Build history of the part. All positions in model axes, mm. Face numbers are marked on the shaded views. A direction names the side the tool comes from. Give positions to 0.01 mm unless a question says otherwise; leave off trailing zeros. Loops run counter-clockwise (first coordinate to the right, second up) from the corner with the lowest first, then second, coordinate; pieces in that order, holes last. Notation, with made-up numbers: M 8,89 L 45,89 A23 ccw 45,100 Z; hole C 16.25,69 d1. An arc over 180 degrees is marked long. Answer in a Markdown table with one row per item. Add a question column.
```python
from build123d import *

# Parameters (mm, degrees)
SKETCH_R        = 2.78
SKETCH_R_2      = 1
PAD_DEPTH       = 1.8
SKETCH001_W     = 10
SKETCH001_H     = 60
PAD001_DEPTH    = 1.8
SKETCH002_W     = 10
SKETCH002_H     = 1.8
PAD002_DEPTH    = 25
SKETCH003_R     = 1.5
POCKET_DEPTH    = 45.701
SKETCH004_R     = 0.5
POCKET001_DEPTH = 26.801


with BuildPart() as part:
    # Sketch → Pad (new body)
    with BuildSketch(Plane.XY):
        with BuildLine():
            ThreePointArc((0, 5), (-5, 0), (0, -5))
            Line((0, -5), (20, -5))
            Line((20, 5), (20, -5))
            Line((0, 5), (20, 5))
        make_face()
        Circle(SKETCH_R, mode=Mode.SUBTRACT)
        with Locations((7.3, 0)):
            Circle(SKETCH_R_2, mode=Mode.SUBTRACT)
        with Locations((13.3, 0)):
            Circle(SKETCH_R_2, mode=Mode.SUBTRACT)
    extrude(amount=PAD_DEPTH)

    # Sketch001 → Pad001 (new body)
    with BuildSketch(Plane.YZ.offset(20)):
        with Locations((0, -21.3)):
            Rectangle(SKETCH001_W, SKETCH001_H)
    extrude(amount=PAD001_DEPTH)

    # Sketch002 → Pad002 (new body)
    with BuildSketch(Plane(origin=(20, 0, 0), x_dir=(0, -1, 0), z_dir=(-1, 0, 0))):
        with Locations((0, -36.1)):
            Rectangle(SKETCH002_W, SKETCH002_H)
    extrude(amount=PAD002_DEPTH)

    # Sketch003 → Pocket (cut, through all)
    with BuildSketch(Plane(origin=(0, 0, -37), x_dir=(1, 0, 0), z_dir=(0, 0, -1))):
        Circle(SKETCH003_R)
    extrude(amount=-POCKET_DEPTH, mode=Mode.SUBTRACT)

    # Sketch004 → Pocket001 (cut, through all)
    with BuildSketch(Plane.YZ.offset(21.8)):
        with Locations((2.1, -42.3)):
            Circle(SKETCH004_R)
        with Locations((-1.6, 6.2)):
            Circle(SKETCH004_R)
    extrude(amount=-POCKET001_DEPTH, mode=Mode.SUBTRACT)


solid = part.part
```
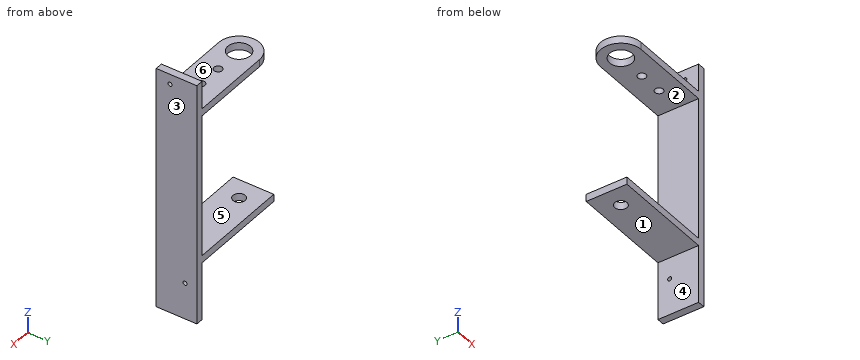
(1) Wall check: line 1 (Z direction, x = 15.5, y = 4); line 2 (Y direction, x = 13.3, z = 0.65); line 3 (Y direction, x = 0, z = -35.8). Give the ranges that are in metal, low to high.
(2) Pull direction Z, two halves, no side cores. Call the marked faces 1, 2 and 3: +Z half, -Z half, draft (parallel to the pull), parting line (faces both ways), or undercut.
(3) Slice it at C-C, the plane y = 3.5. Give the cut face in (x, z).
(4) Slice it at B-B, the plane x = 7.3. Give the cut face in (y, z), then the cut area to 3 significant figures.
(5) Slice it at A-A, the plane x = 10.75. Give the cut face in (y, z), then the cut area to 3 significant figures.
(6) Pin check, flat tips, straight feed: pin 1 (3.5 mm diameter, centred on x = 0, y = 0, fed in from -Z); pin 2 (4.5 mm diameter, centred on x = 0, y = 0, fed in from +Z); pin 3 (5 mm diameter, centred on y = 2, z = -16.5, fed in from -X); pin 4 (2 mm diameter, centred on x = 7, z = -34, fed in from -Y). Stop position of each tip, or through.
(7) Slice it at D-D, the plane z = -13.5. Give the cut face in (x, y), then the cut area to 3 significant figures.
(8) Tool access for the marked faces 4, 5 and 6: list every direction of +Z, -Z, +X, -X, +Y, -Y with a clear straight run to the whole face (end or side of a thin tool).
Solution:
| question | item | result |
|---|---|---|
| 1 | line 1 | -37 to -35.2, 0 to 1.8 |
| 1 | line 2 | -5 to -1, 1 to 5 |
| 1 | line 3 | -5 to -1.5, 1.5 to 5 |
| 2 | face 1 | -Z half |
| 2 | face 2 | undercut |
| 2 | face 3 | draft |
| 3 | outline | M -5,-37 L 20,-37 L 20,-51.3 L 21.8,-51.3 L 21.8,8.7 L 20,8.7 L 20,1.8 L -3.57,1.8 L -3.57,0 L 20,0 L 20,-35.2 L -5,-35.2 Z |
| 4 | outline | M -5,-37 L 5,-37 L 5,-35.2 L -5,-35.2 Z; M -5,0 L -1,0 L -1,1.8 L -5,1.8 Z; M 1,0 L 5,0 L 5,1.8 L 1,1.8 Z |
| 4 | area | 32.4 mm^2 |
| 5 | outline | M -5,-37 L 5,-37 L 5,-35.2 L -5,-35.2 Z; M -5,0 L 5,0 L 5,1.8 L -5,1.8 Z |
| 5 | area | 36.0 mm^2 |
| 6 | pin 1 | z = -37 |
| 6 | pin 2 | z = -35.2 |
| 6 | pin 3 | x = 20 |
| 6 | pin 4 | through |
| 7 | outline | M 20,-5 L 21.8,-5 L 21.8,5 L 20,5 Z |
| 7 | area | 18.0 mm^2 |
| 8 | face 4 | -Z, -X, +Y, -Y |
| 8 | face 5 | -X, +Y, -Y |
| 8 | face 6 | +Z, -X, +Y, -Y |
